```python
from build123d import *

# Parameters (mm, degrees)
SKETCH1_W            = 32.64025
SKETCH1_H            = 35.56
SKETCH1_R            = 2.1
BOSS_EXTRUDE2_DEPTH  = 3.175
BOSS_EXTRUDE3_DEPTH  = 1.5875
SKETCH4_W            = 11.385
SKETCH4_H            = 16.825
SKETCH4_R            = 2.45
BOSS_EXTRUDE4_DEPTH  = 1.5875
MIRROR2_COPY_1_DEPTH = 1.5875
FILLET1_R            = 0.762
FILLET2_R            = 0.762
FILLET6_R            = 0.762
FILLET7_R            = 0.762


with BuildPart() as part:
    # Sketch1 → Boss-Extrude2 (new body)
    with BuildSketch(Plane(origin=(0, 0, 0), x_dir=(1, 0, 0), z_dir=(0, 1, 0))):
        with Locations((24.319875, 0)):
            Rectangle(SKETCH1_W, SKETCH1_H)
        with Locations((35.71875, 12.7)):
            Circle(SKETCH1_R, mode=Mode.SUBTRACT)
        with Locations((35.71875, -12.7)):
            Circle(SKETCH1_R, mode=Mode.SUBTRACT)
    extrude(amount=BOSS_EXTRUDE2_DEPTH)

    # Sketch2 → Boss-Extrude3 (add)
    with BuildSketch(Plane.XY.offset(17.78)):
        with BuildLine():
            Line((17.798889871, 19.185782349), (39.830221584, 6.805062799))
            ThreePointArc((39.830221584, 6.805062799), (40.422680511, 6.222841365), (40.64, 5.421117212))
            Line((40.64, 5.421117212), (40.64, 3.175))
            Line((40.64, 3.175), (7.99975, 3.175))
            Line((7.99975, 3.175), (7.99975, 20))
            Line((7.99975, 20), (11.5875, 20))
            Line((11.5875, 20), (14.688003537, 20))
            ThreePointArc((14.688003537, 20), (16.295840918, 19.793074064), (17.798889871, 19.185782349))
        make_face()
    boss_extrude3 = extrude(amount=-BOSS_EXTRUDE3_DEPTH)

    # Mirror1: Boss-Extrude3 across plane
    add(boss_extrude3.mirror(Plane.XY.offset(10.5)))

    # Sketch4 → Boss-Extrude4 (add)
    with BuildSketch(Plane.ZY.offset(-7.99975)):
        with Locations((10.5, 11.5875)):
            Rectangle(SKETCH4_W, SKETCH4_H)
        with Locations((10.5, 10)):
            Circle(SKETCH4_R, mode=Mode.SUBTRACT)
    boss_extrude4 = extrude(amount=-BOSS_EXTRUDE4_DEPTH)

    # Mirror2: Boss-Extrude3, Boss-Extrude4 across plane
    add(boss_extrude3.mirror(Plane.XY))
    add(boss_extrude4.mirror(Plane.XY))

    # Mirror2 copy 1 sketch → Mirror2 copy 1 (add)
    with BuildSketch(Plane.XY.offset(-3.22)):
        with BuildLine():
            Line((17.798889871, 19.185782349), (39.830221584, 6.805062799))
            ThreePointArc((39.830221584, 6.805062799), (40.422680511, 6.222841365), (40.64, 5.421117212))
            Line((40.64, 5.421117212), (40.64, 3.175))
            Line((40.64, 3.175), (7.99975, 3.175))
            Line((7.99975, 3.175), (7.99975, 20))
            Line((7.99975, 20), (11.5875, 20))
            Line((11.5875, 20), (14.688003537, 20))
            ThreePointArc((14.688003537, 20), (16.295840918, 19.793074064), (17.798889871, 19.185782349))
        make_face()
    extrude(amount=-MIRROR2_COPY_1_DEPTH)

    # Fillet1
    fillet1_edges = [part.edges().sort_by_distance(p)[0] for p in [
        (9.58725, 11.5875, 4.8075),
    ]]
    fillet(fillet1_edges, radius=FILLET1_R)

    # Fillet2
    fillet2_edges = [part.edges().sort_by_distance(p)[0] for p in [
        (9.58725, 11.5875, 16.1925),
    ]]
    fillet(fillet2_edges, radius=FILLET2_R)

    # Fillet6
    fillet6_edges = [part.edges().sort_by_distance(p)[0] for p in [
        (24.319875, 3.175, 3.22),
    ]]
    fillet(fillet6_edges, radius=FILLET6_R)

    # Fillet7
    fillet7_edges = [part.edges().sort_by_distance(p)[0] for p in [
        (24.319875, 3.175, -3.22),
        (25.113625, 3.175, -4.8075),
        (25.113625, 3.175, -16.1925),
        (9.58725, 11.5875, -16.1925),
        (9.58725, 11.5875, -4.8075),
        (9.58725, 3.175, -10.5),
        (25.494625, 3.175, 4.8075),
        (9.58725, 3.175, 10.5),
        (9.810434633, 3.175, 5.030684633),
        (25.494625, 3.175, 16.1925),
        (9.810434633, 3.175, 15.969315367),
    ]]
    fillet(fillet7_edges, radius=FILLET7_R)


solid = part.part
```
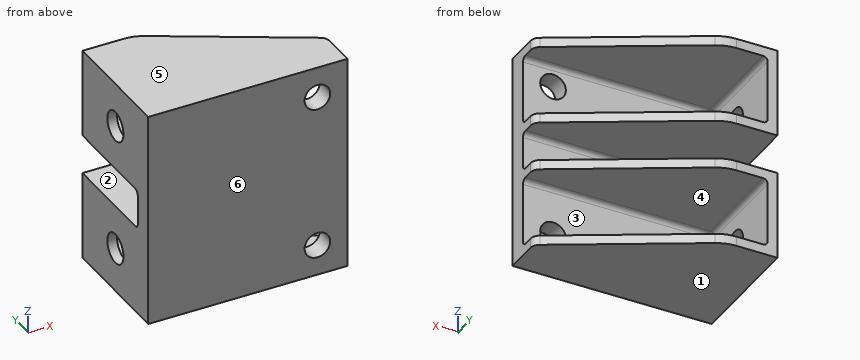
Geometry check sheet. Reference: the model listing, model coordinates, mm. Face numbers are marked on the shaded views. A direction names the side the tool comes from. Coordinates: 2 decimals unless noted, no trailing zeros. Loops run counter-clockwise (first coordinate to the right, second up) from the corner with the lowest first, then second, coordinate; pieces in that order, holes last. Notation, with made-up numbers: (6, 6.5) -> (22, 6.5) arc R9 ccw to (22, 17.5) -> close; hole circle Ø7 at (8.5, -18.5). An arc over 180 degrees is marked (long way). Put each result on its own line as item: value.
1) Cross-section at D-D on x = 35.5. Count the separate pieces of the cut face and the enclosed holes in it, plus the area to 3 significant figures.
Result set:
separate pieces: 3
enclosed holes: 0
area: 126 mm^2
2) Release check for a two-part mould opening along Z. For the marked faces 4, 5 and 6 record: released by +Z, released by -Z, zero draft, split by the parting line, or undercut.
Result set:
face 4: undercut
face 5: released by +Z
face 6: zero draft
3) Tool access check on the marked faces 1, 2 and 3. Record the directions out of +Z, -Z, +X, -X, +Y, -Y that give a thin tool (end or side, any length) a straight path to the whole face; none if there is none.
Result set:
face 1: -Z, +X, -X, +Y, -Y
face 2: +X, -X, +Y
face 3: +X, +Y
4) Thickness scan on line 1 (Z direction, x = 18, y = 16); line 2 (Y direction, x = 13, z = 7) (3 decimals); line 3 (X direction, y = 16.75, z = -9). Record the ranges inside material, lowest first.
Result set:
line 1: z = -17.78 to -16.19, -4.81 to -3.22, 3.22 to 4.81, 16.19 to 17.78
line 2: y = 0 to 3.175
line 3: x = 8 to 9.59
5) Cross-section at A-A on y = 16.25. Record the boundary of the cut face in (x, z), plus the area to 3 significant figures.
Result set:
outline: (8, -17.78) -> (23.02, -17.78) -> (23.02, -16.19) -> (10.35, -16.19) arc R0.76 cw to (9.59, -15.43) -> (9.59, -5.57) arc R0.76 cw to (10.35, -4.81) -> (23.02, -4.81) -> (23.02, -3.22) -> (8, -3.22) -> close; (8, 3.22) -> (23.02, 3.22) -> (23.02, 4.81) -> (10.35, 4.81) arc R0.76 cw to (9.59, 5.57) -> (9.59, 15.43) arc R0.76 cw to (10.35, 16.19) -> (23.02, 16.19) -> (23.02, 17.78) -> (8, 17.78) -> close
area: 132 mm^2
6) Cross-section at C-C on x = 13. Record the boundary of the cut face in (y, z) (1 decimal).
Result set:
outline: (0, -17.8) -> (20, -17.8) -> (20, -16.2) -> (3.9, -16.2) arc R0.8 cw to (3.2, -15.4) -> (3.2, -5.6) arc R0.8 cw to (3.9, -4.8) -> (20, -4.8) -> (20, -3.2) -> (3.9, -3.2) arc R0.8 cw to (3.2, -2.5) -> (3.2, 2.5) arc R0.8 cw to (3.9, 3.2) -> (20, 3.2) -> (20, 4.8) -> (3.9, 4.8) arc R0.8 cw to (3.2, 5.6) -> (3.2, 15.4) arc R0.8 cw to (3.9, 16.2) -> (20, 16.2) -> (20, 17.8) -> (0, 17.8) -> close
7) Gauge pin test, flat ends, axial feed: pin 1 Ø3 at (y, z) = (14, 10) entering from +X; pin 2 Ø11 at (x, z) = (33, -10.5) entering from +Y; pin 3 Ø3 at (x, z) = (25.5, 9.5) entering from +Y (3 decimals). Record the tip position at first contact, or that the pin passes through.
Result set:
pin 1: stops at x = 9.59
pin 2: stops at y = 3.43
pin 3: stops at y = 3.175
8) Cross-section at B-B on z = 9.5. Record the boundary of the cut face in (x, y) (3 decimals).
Result set:
outline: (8, 0) -> (40.64, 0) -> (40.64, 3.175) -> (10.349, 3.175) arc R0.762 cw to (9.587, 3.937) -> (9.587, 7.763) -> (8, 7.763) -> close; (8, 12.237) -> (9.587, 12.237) -> (9.587, 20) -> (8, 20) -> close
